The model under review builds one solid part; all positions refer to its coordinate system, in mm. Face numbers are marked on the shaded views. A direction names the side the tool comes from. Round coordinates to 2 decimals unless told otherwise and drop trailing zeros. Write each loop counter-clockwise with the first axis right and the second up, starting at its lowest first coordinate (ties: lowest second). Pieces come first, ordered by that corner, then holes. Notation, with made-up numbers: (46.5, -25) -> (87.5, -25) arc R33 ccw to (87.5, 11) -> close; hole circle Ø9 at (-34, -28). An arc over 180 degrees is marked (long way). Answer in a Markdown table with one row per item. Add a question column.
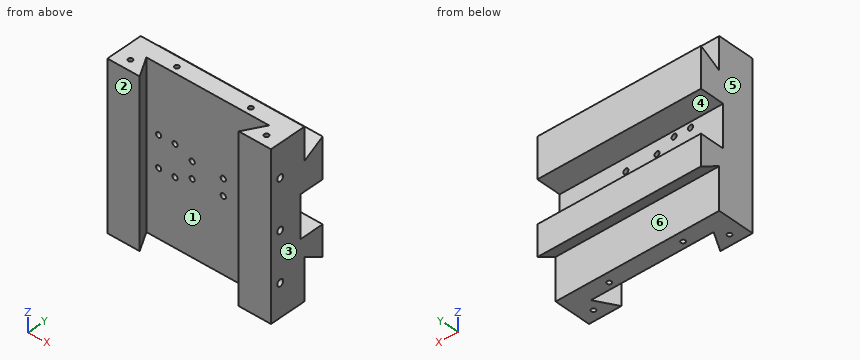
```python
from build123d import *

# Parameters (mm, degrees)
X_CARRIAGE_EXTRUDE_DEPTH                 = 63.5
Y_GUIDE_CUT_EXTRUDE_DEPTH                = 63.5
F_8_32_TAPPED_HOLE1_D                    = 3.4544
F_8_32_TAPPED_HOLE1_DEPTH                = 12.3444
F_8_32_TAPPED_HOLE1_TIP                  = 1.037806461
F_8_32_TAPPED_HOLE2_D                    = 3.4544
F_8_32_TAPPED_HOLE2_DEPTH                = 12.446
F_8_32_TAPPED_HOLE2_TIP                  = 1.037806461
SKETCH8_W                                = 2.5527
SKETCH8_H                                = 63.5
GIB_SCREW_1_4_20_TAPPED_HOLE1_AT_2_COUNT = 2
GIB_SCREW_1_4_20_TAPPED_HOLE1_AT_2_PITCH = 38.1
GIB_SCREW_1_4_20_TAPPED_HOLE1_AT_3_COUNT = 2
GIB_SCREW_1_4_20_TAPPED_HOLE1_AT_3_PITCH = 76.2
F_10_32_TAPPED_HOLE1_D                   = 4.0386
F_10_32_TAPPED_HOLE1_DEPTH               = 9.271


with BuildPart() as part:
    # female-dovetail-profile → x-carriage-extrude (new, symmetric)
    with BuildSketch(Plane.XY):
        Polygon((-47.625, 15.875), (-40.292651581, 15.875), (-16.056336319, 15.875), (16.056336319, 15.875), (47.625, 15.875), (38.459564477, 0), (63.5, 0), (63.5, 31.75), (63.5, 44.45), (-63.5, 44.45), (-63.5, 31.75), (-63.5, 0), (-38.459564477, 0), align=None)
    extrude(amount=X_CARRIAGE_EXTRUDE_DEPTH, both=True)

    # male-dovetail-shoulder-profile → y-guide-cut-extrude (cut, symmetric)
    with BuildSketch(Plane(origin=(0, 0, 0), x_dir=(0, 0, -1), z_dir=(1, 0, 0))):
        Polygon((63.5, 28.575), (38.459564477, 28.575), (31.127216058, 28.575), (40.146004613, 44.196), (16.310336319, 44.196), (16.310336319, 25.146), (-16.310336319, 25.146), (-16.310336319, 44.196), (-47.478353032, 44.196), (-38.459564477, 28.575), (-63.5, 28.575), (-63.5, 44.45), (63.5, 44.45), align=None)
    extrude(amount=Y_GUIDE_CUT_EXTRUDE_DEPTH, both=True, mode=Mode.SUBTRACT)

    # #8-32 Tapped Hole1
    with Locations(Plane(origin=(0, -15.875, 63.5), x_dir=(1, 0, 0), z_dir=(0, 0, 1))):
        with Locations((-52.832, 23.8125), (-28.702, 36.957), (28.702, 36.957), (52.832, 23.8125)):
            Hole(F_8_32_TAPPED_HOLE1_D / 2, depth=F_8_32_TAPPED_HOLE1_DEPTH)
            with Locations((0, 0, -(F_8_32_TAPPED_HOLE1_DEPTH + F_8_32_TAPPED_HOLE1_TIP / 2))):  # 118° drill point
                Cone(0, F_8_32_TAPPED_HOLE1_D / 2, F_8_32_TAPPED_HOLE1_TIP, mode=Mode.SUBTRACT)

    # #8-32 Tapped Hole2
    with Locations(Plane(origin=(0, -15.875, -63.5), x_dir=(-1, 0, 0), z_dir=(0, 0, -1))):
        with Locations((-52.832, 23.8125), (-28.702, 36.957), (28.702, 36.957), (52.832, 23.8125)):
            Hole(F_8_32_TAPPED_HOLE2_D / 2, depth=F_8_32_TAPPED_HOLE2_DEPTH)
            with Locations((0, 0, -(F_8_32_TAPPED_HOLE2_DEPTH + F_8_32_TAPPED_HOLE2_TIP / 2))):  # 118° drill point
                Cone(0, F_8_32_TAPPED_HOLE2_D / 2, F_8_32_TAPPED_HOLE2_TIP, mode=Mode.SUBTRACT)

    # Sketch8 → gib screw 1/4-20 Tapped Hole1 (revolve, cut)
    with BuildSketch(Plane(origin=(0, 7.9375, 38.1), x_dir=(0, 0, 1), z_dir=(0, 1, 0))):
        with Locations((1.27635, 31.75)):
            Rectangle(SKETCH8_W, SKETCH8_H)
    gib_screw_1_4_20_tapped_hole1 = revolve(axis=Axis((-6.35, 7.9375, 38.1), (1, 0, 0)), mode=Mode.SUBTRACT)

    # gib screw 1/4-20 Tapped Hole1 at 2: gib screw 1/4-20 Tapped Hole1 ×2
    with Locations(*[(0, 0, -i * GIB_SCREW_1_4_20_TAPPED_HOLE1_AT_2_PITCH) for i in range(1, GIB_SCREW_1_4_20_TAPPED_HOLE1_AT_2_COUNT)]):
        add(gib_screw_1_4_20_tapped_hole1, mode=Mode.SUBTRACT)

    # gib screw 1/4-20 Tapped Hole1 at 3: gib screw 1/4-20 Tapped Hole1 ×2
    with Locations(*[(0, 0, -i * GIB_SCREW_1_4_20_TAPPED_HOLE1_AT_3_PITCH) for i in range(1, GIB_SCREW_1_4_20_TAPPED_HOLE1_AT_3_COUNT)]):
        add(gib_screw_1_4_20_tapped_hole1, mode=Mode.SUBTRACT)

    # #10-32 Tapped Hole1
    with Locations(Plane(origin=(0, 25.146, 0), x_dir=(1, 0, 0), z_dir=(0, 1, 0))):
        with Locations((-38.1, 12.065), (-38.1, -12.065), (-12.065, 6.35), (-25.4, 12.065), (-25.4, -12.065), (12.065, 6.35), (12.065, -6.35), (-12.065, -6.35)):
            Hole(F_10_32_TAPPED_HOLE1_D / 2, depth=F_10_32_TAPPED_HOLE1_DEPTH)


solid = part.part
```
1. Add section B-B on y = 27. Write out the cut boundary in (x, z), plus the area to 3 significant figures.
2. Tool access review of the marked faces 4, 5 and 6: name each direction out of +Z, -Z, +X, -X, +Y, -Y from which nothing blocks a thin tool from reaching the whole face with its end or side.
3. Add section C-C on z = 1. Write out the cut boundary in (x, y) (3 decimals).
4. For L1, parallel to Z at x = -38, y = 21; L2, parallel to Y at x = 57.5, z = -38.1 (3 decimals); L3, parallel to Z at x = -55, y = 27.5, list the stretches that pass through material, from the lowest coordinate up.
5. Add section A-A on x = -25.4. Write out the cut boundary in (y, z) (3 decimals).
6. Add section D-D on x = 33. Write out the cut boundary in (y, z) (3 decimals).
7. Mouldability with a two-part tool opening along Y and no side actions: class the marked faces 1, 2 and 3 as pulls with the +Y half, pulls with the -Y half, needs draft (parallel to the pull), parting line crosses it, or undercut.
8. Insertion check: pin 1 Ø2 at (x, y) = (52.83, 7.94) entering from +Z; pin 2 Ø5.5 at (x, z) = (-12.065, -6.35) entering from -Y (3 decimals); pin 3 Ø2.5 at (x, z) = (-25.4, -12.065) entering from +Y; pin 4 Ø3 at (x, y) = (52.83, 7.94) entering from -Z. Each pin has a flat end and moves straight along its axis. Give the tip position at first contact, or say it passes through.
Filled in:
| question | item | result |
|---|---|---|
| 1 | outline | (-63.5, -63.5) -> (63.5, -63.5) -> (63.5, -16.31) -> (-63.5, -16.31) -> close; (-63.5, 16.31) -> (63.5, 16.31) -> (63.5, 63.5) -> (-63.5, 63.5) -> close |
| 1 | area | 12,000 mm² |
| 2 | face 4 | +X, -X, +Y |
| 2 | face 5 | +Z, -Z, -X, +Y, -Y |
| 2 | face 6 | -Z, +X, -X |
| 3 | outline | (-63.5, 0) -> (-38.46, 0) -> (-47.625, 15.875) -> (47.625, 15.875) -> (44.398, 10.286) -> (63.5, 10.286) -> (63.5, 25.146) -> (-63.5, 25.146) -> close; (38.46, 0) -> (63.5, 0) -> (63.5, 5.589) -> (41.686, 5.589) -> close |
| 4 | L1 | -63.5 to -14.08, -10.05 to 10.05, 14.08 to 63.5 |
| 4 | L2 | 0 to 5.385, 10.49 to 28.575, 40.652 to 44.196 |
| 4 | L3 | -63.5 to -16.31, 16.31 to 63.5 |
| 5 | outline | (15.875, -63.5) -> (28.575, -63.5) -> (28.575, -31.127) -> (44.196, -40.146) -> (44.196, -16.31) -> (25.146, -16.31) -> (25.146, -14.084) -> (15.875, -14.084) -> close; (15.875, -10.046) -> (25.146, -10.046) -> (25.146, 10.046) -> (15.875, 10.046) -> close; (15.875, 14.084) -> (25.146, 14.084) -> (25.146, 16.31) -> (44.196, 16.31) -> (44.196, 47.478) -> (28.575, 38.46) -> (28.575, 63.5) -> (15.875, 63.5) -> close |
| 6 | outline | (15.875, -63.5) -> (28.575, -63.5) -> (28.575, -31.127) -> (44.196, -40.146) -> (44.196, -16.31) -> (25.146, -16.31) -> (25.146, 16.31) -> (44.196, 16.31) -> (44.196, 47.478) -> (28.575, 38.46) -> (28.575, 63.5) -> (15.875, 63.5) -> close |
| 7 | face 1 | undercut |
| 7 | face 2 | pulls with the -Y half |
| 7 | face 3 | needs draft |
| 8 | pin 1 | z = 50.72 |
| 8 | pin 2 | y = 15.875 |
| 8 | pin 3 | through |
| 8 | pin 4 | z = -50.92 |
